from build123d import *

# Parameters (mm, degrees)
F0_R     = 2.5
F1_DEPTH = 4
F2_SIZE  = 1.99999
F3_W     = 3.2302876376
F3_H     = 15.0867640845
F4_DEPTH = 4


# Not quite as in the source:
# - a fillet or chamfer is up to 0.001 mm smaller than in the source, because OpenCascade refuses the exact size


with BuildPart() as f1:
    # F0 (on Top) → F1 (new body)
    with BuildSketch(Plane.XY):
        with BuildLine():
            ThreePointArc((-6.116279643, 38.6264544598), (-16.116279643, 28.6264544598), (-26.116279643, 38.6264544598))
            Line((-26.116279643, 38.6264544598), (-26.116279643, 6.1264544598))
            Line((-26.116279643, 6.1264544598), (-16.116279643, -3.8735455402))
            Line((-16.116279643, -3.8735455402), (-13.616279643, -6.3735455402))
            Line((-13.616279643, -6.3735455402), (-13.616279643, -12.0434185212))
            Line((-13.616279643, -12.0434185212), (-13.616279643, -16.3735455402))
            Line((-13.616279643, -16.3735455402), (-13.616279643, -20.7036725591))
            ThreePointArc((-13.616279643, -20.7036725591), (-18.616279643, -20.7036725591), (-21.116279643, -16.3735455402))
            Line((-21.116279643, -16.3735455402), (-21.116279643, -11.3735455402))
            Line((-21.116279643, -11.3735455402), (-26.116279643, -6.3735455402))
            Line((-26.116279643, -6.3735455402), (-26.116279643, -16.3735455402))
            ThreePointArc((-26.116279643, -16.3735455402), (-16.116279643, -26.3735455402), (-6.116279643, -16.3735455402))
            Line((-6.116279643, -16.3735455402), (-6.116279643, 38.6264544598))
        make_face()
        with BuildLine():
            ThreePointArc((-6.116279643, 38.6264544598), (-16.116279643, 48.6264544598), (-26.116279643, 38.6264544598))
            ThreePointArc((-26.116279643, 38.6264544598), (-16.116279643, 28.6264544598), (-6.116279643, 38.6264544598))
        make_face()
        with Locations((-16.116279643, 43.6264544598)):
            Circle(F0_R, mode=Mode.SUBTRACT)
        with BuildLine():
            Line((-13.616279643, -20.7036725591), (-13.616279643, -16.3735455402))
            ThreePointArc((-13.616279643, -16.3735455402), (-16.116279643, -18.8735455402), (-18.616279643, -16.3735455402))
            Line((-18.616279643, -16.3735455402), (-18.616279643, -13.8735455402))
            Line((-18.616279643, -13.8735455402), (-21.116279643, -11.3735455402))
            Line((-21.116279643, -11.3735455402), (-21.116279643, -16.3735455402))
            ThreePointArc((-21.116279643, -16.3735455402), (-18.616279643, -20.7036725591), (-13.616279643, -20.7036725591))
        make_face()
    extrude(amount=F1_DEPTH)

    # F2 (size 2 in the source; OpenCascade refuses exactly that, so slightly less here)
    f2_edges = [f1.edges().sort_by_distance(p)[0] for p in [
        (-16.11628, -18.873546, 4),
        (-18.61628, -15.123546, 4),
        (-16.11628, -18.873546, 0),
    ]]
    chamfer(f2_edges, length=F2_SIZE)

    # F3 (on face) → F4 (join)
    with BuildSketch(Plane.XY.offset(4)):
        with Locations((-12.0011358242, -13.9169275824)):
            Rectangle(F3_W, F3_H)
    extrude(amount=-F4_DEPTH)


solid = f1.part
For this review, take the finished solid that the model builds, in its own axes (mm). A direction names the side the tool comes from. Round coordinates to 2 decimals unless told otherwise and drop trailing zeros. Write each loop counter-clockwise with the first axis right and the second up, starting at its lowest first coordinate (ties: lowest second). Pieces come first, ordered by that corner, then holes. Notation, with made-up numbers: M -15.5,35.25 L 29.5,35.25 A26 cw 29.5,66.25 Z; hole C -21.75,12 d7. An arc over 180 degrees is marked long. Write item = value, one per line. Start each with the question number.
(1) We need section A-A (z = 1.3). Give the boundary of the cut face in (x, y).
(2) We need section D-D (x = -8.5). Give the boundary of the cut face in (y, z), then the cut area to 3 significant figures.
(3) For line 1 along Y through (x, z) = (-16.75, 0.2); line 2 along Y through (x, z) = (-15.5, 0.65); line 3 along Y through (x, z) = (-21.25, 0.9), list the stretches that pass through material, from the lowest coordinate up.
(4) We need section B-B (x = -14.75). Give the number of separate pieces and of enclosed holes in the cut face, then the cut area to 3 significant figures.
(5) We need section C-C (y = -5). Give the boundary of the cut face in (x, z), then the cut area to 3 significant figures.
(6) For faces 1 (the face through (-23.15, -9.34, 1.97)), 2 (the face through (-19.95, -0.04, 1.97)), 3 (the face through (-17.1, -19.28, 1.43)), 4 (the face through (-17.1, -19.28, 2.57)), list the 3-axis set-ups (+Z, -Z, +X, -X, +Y, -Y) from which the entire face can be reached by the end or side of a thin tool; tool diameter is ignored.
(7) The part is to be moulded in two halves that separate along Y. For faces 5 (the face through (-16.34, -26.37, 1.97)), 6 (the face through (-19.63, -14.655, 3.014)), 7 (the face through (-26.116, -11, 2)), 8 (the face through (-15.896, 48.624, 1.972)), say which applies: +Y half, -Y half, draft (parallel to the pull), parting line (faces both ways), or undercut.
(8) Clearance check with a flat-ended pin moving along its axis: pin 1 Ø4 at (x, y) = (-16, -14) entering from +Z. State where the tip first meets the part, or that it passes through.
Results found:
q1.outline = M -26.12,-16.37 A10 ccw -6.12,-16.37 L -6.12,38.63 A10 ccw -26.12,38.63 L -26.12,6.13 L -13.62,-6.37 L -13.62,-18.37 A3.2 cw -19.32,-16.37 L -19.32,-13.17 L -26.12,-6.37 Z; hole C -16.12,43.63 d5
q2.outline = M -22.85,0 L 45.11,0 L 45.11,4 L -22.85,4 Z
q2.area = 272 mm²
q3.line_1 = -26.35 to -20.63, -3.24 to 41.21, 46.04 to 48.61
q3.line_2 = -26.35 to -20.17, -4.49 to 41.2, 46.05 to 48.61
q3.line_3 = -24.96 to -11.24, 1.26 to 47.21
q4.separate_pieces = 3
q4.enclosed_holes = 0
q4.area = 225 mm²
q5.outline = M -14.99,0 L -6.12,0 L -6.12,4 L -14.99,4 Z
q5.area = 35.5 mm²
q6.face_1 = +Z, -Z
q6.face_2 = +Z, -Z, -X
q6.face_3 = -Z
q6.face_4 = +Z
q7.face_5 = -Y half
q7.face_6 = undercut
q7.face_7 = draft
q7.face_8 = +Y half
q8.pin_1 = through
